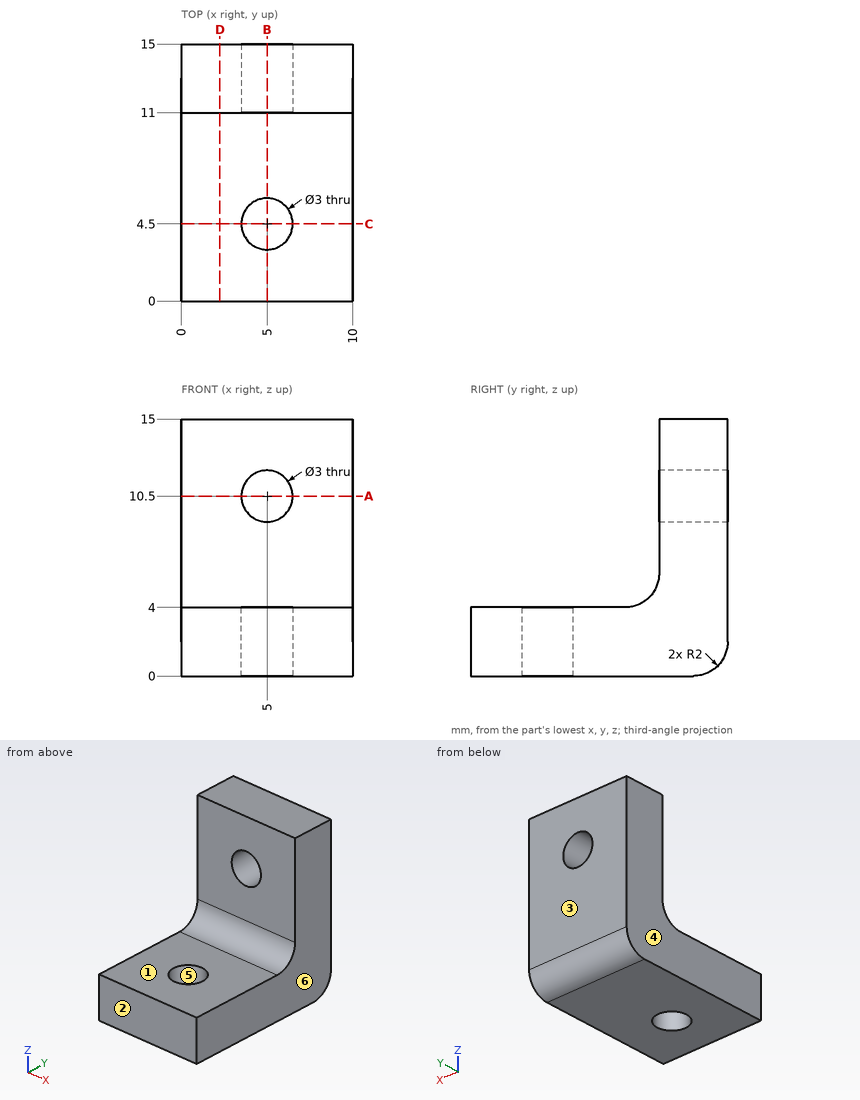
The drawing under review shows one solid part. Ordinate dimensions are in mm from its lowest x, y, z. A direction names the side the tool comes from. Give positions to 0.01 mm unless a question says otherwise; leave off trailing zeros. Write each loop counter-clockwise with the first axis right and the second up, starting at its lowest first coordinate (ties: lowest second). Pieces come first, ordered by that corner, then holes.
1. Wall thickness on L1, parallel to Y at x = 5, z = 2.2; L2, parallel to X at y = 12.75, z = 10.5; L3, parallel to Y at x = 9.5, z = 14.25: over which ranges is each line inside the solid? List them lowest first.
2. Draft analysis for pull direction X (two halves, no side actions). For the marked faces 3, 4, 5 and 6, state which applies: +X half, -X half, draft (parallel to the pull), parting line (faces both ways), or undercut.
3. For P1, Ø4.5, axis at x = 7, y = 3.5, coming from the +Z side; P2, Ø2.5, axis at x = 7, z = 8.5, coming from the -Y side, all flat-tipped, find the tip position at first contact; note any pin that passes through.
4. Add section D-D, the plane x = 2.25. Write out the cut boundary in (y, z), plus the area to 3 significant figures.
5. Add section B-B, the plane x = 5. Write out the cut boundary in (y, z), plus the area to 3 significant figures.
6. Add section A-A, the plane z = 10.5. Write out the cut boundary in (x, y).
7. Tool access review of the marked faces 1 and 2: name each direction out of +Z, -Z, +X, -X, +Y, -Y from which nothing blocks a thin tool from reaching the whole face with its end or side.
8. Add section C-C, the plane y = 4.5. Write out the cut boundary in (x, z).
Worked answers:
1. L1: y = 0 to 3, 6 to 15
1. L2: x = 0 to 3.5, 6.5 to 10
1. L3: y = 11 to 15
2. face 3: draft
2. face 4: -X half
2. face 5: undercut
2. face 6: +X half
3. P1: stops at z = 4
3. P2: stops at y = 11
4. outline: (0, 0) - (13, 0) arc R2 ccw to (15, 2) - (15, 15) - (11, 15) - (11, 6) arc R2 cw to (9, 4) - (0, 4) - close
4. area: 104 mm2
5. outline: (0, 0) - (3, 0) - (3, 4) - (0, 4) - close; (6, 0) - (13, 0) arc R2 ccw to (15, 2) - (15, 9) - (11, 9) - (11, 6) arc R2 cw to (9, 4) - (6, 4) - close; (11, 12) - (15, 12) - (15, 15) - (11, 15) - close
5. area: 80.0 mm2
6. outline: (0, 11) - (3.5, 11) - (3.5, 15) - (0, 15) - close; (6.5, 11) - (10, 11) - (10, 15) - (6.5, 15) - close
7. face 1: +Z, +X, -X, -Y
7. face 2: +Z, -Z, +X, -X, -Y
8. outline: (0, 0) - (3.5, 0) - (3.5, 4) - (0, 4) - close; (6.5, 0) - (10, 0) - (10, 4) - (6.5, 4) - close
